from build123d import *

# Parameters (mm, degrees)
F0_W     = 35.56
F0_H     = 37.1792408654
F1_DEPTH = 17.4625
F3_DEPTH = 4.7625
F4_R     = 5.08
F5_R     = 5.08


# Not quite as in the source:
# - a length typed as a fraction of an inch, garbled in the dataset ("3 / 203.2 mm" for 3/8 in), is restored


with BuildPart() as f1:
    # F0 (on Top) → F1 (new body)
    with BuildSketch(Plane.XY):
        Rectangle(F0_W, F0_H)
    extrude(amount=F1_DEPTH)

    # F2 (on face) → F3 (cut)
    with BuildSketch(Plane.XY.offset(17.4625)):
        with BuildLine():
            Line((-12.7, -18.5896204327), (17.78, -18.5896204327))
            Line((17.78, -18.5896204327), (17.78, 13.5096204327))
            Line((17.78, 13.5096204327), (-8.89, 13.5096204327))
            ThreePointArc((-8.89, 13.5096204327), (-15.3940768363, 16.203697269), (-12.7, 9.6996204327))
            Line((-12.7, 9.6996204327), (-12.7, -18.5896204327))
        make_face()
    extrude(amount=-F3_DEPTH, mode=Mode.SUBTRACT)

    # F4
    f4_edges = [f1.edges().sort_by_distance(p)[0] for p in [
        (-12.7, 9.69962, 15.08125),
        (-8.89, 13.50962, 15.08125),
    ]]
    fillet(f4_edges, radius=F4_R)

    # F5
    f5_edges = [f1.edges().sort_by_distance(p)[0] for p in [
        (-17.78, 18.58962, 8.73125),
    ]]
    fillet(f5_edges, radius=F5_R)


solid = f1.part
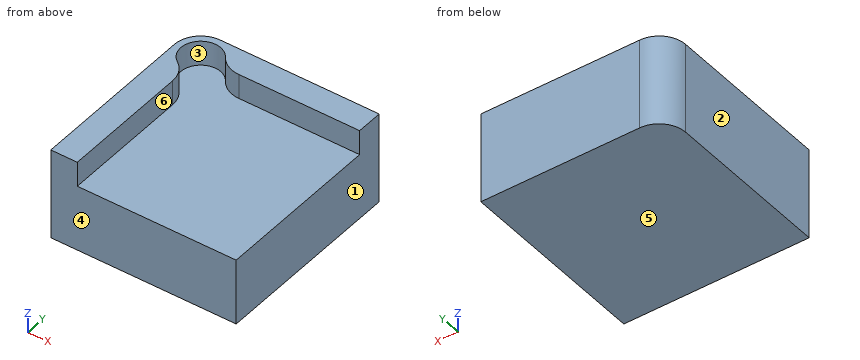
The listing builds one solid part. Answer for the finished solid, in the listing's coordinates (mm). Face numbers are marked on the shaded views. A direction names the side the tool comes from. Round coordinates to 2 decimals unless told otherwise and drop trailing zeros. Write each loop counter-clockwise with the first axis right and the second up, starting at its lowest first coordinate (ties: lowest second). Pieces come first, ordered by that corner, then holes. Notation, with made-up numbers: M 40,-4.75 L 70,-4.75 A12 cw 70,17.25 Z; hole C -19,29 d5. An arc over 180 degrees is marked long. Write each question's results on one line, items separated by ' | '. Start each with the question number.
(1) This flat-tipped pin is pushed along its axis until it touches: P1, Ø5, axis at x = 11.5, z = 16, coming from the -Y side. Where does it stop, or does it pass through?
(2) Find the intervals of material crossed by line 1 (Z direction, x = -8, y = -15.5); line 2 (X direction, y = 5.5, z = 13.5); line 3 (Y direction, x = 13, z = 15.25), in increasing order.
(3) For the marked faces 5 and 6, determine the directions among +Z, -Z, +X, -X, +Y, -Y from which every point of the face is accessible in a straight line to the end or side of a thin tool.
(4) The part is cut by section C-C, the plane y = 14. Write down the section's boundary in (x, z), and give its area (3 significant figures).
(5) Determine the mould class of the marked faces 1, 2, 3 and 4 for opening direction X: +X half, -X half, draft (parallel to the pull), parting line (faces both ways), or undercut.
(6) The part is cut by section A-A, the plane y = 2. Write down the section's boundary in (x, z).
(7) The part is cut by section B-B, the plane x = -14. Write down the section's boundary in (y, z), and give its area (3 significant figures).
Worked answers:
1) P1: stops at y = 13.51
2) line 1: z = 0 to 12.7 | line 2: x = -17.78 to -12.7 | line 3: y = 13.51 to 18.59
3) face 5: -Z, +X, -X, +Y, -Y | face 6: +Z, +X, -Y
4) outline: M -17.76,0 L 17.78,0 L 17.78,17.46 L -7.58,17.46 L -7.58,12.7 L -16.48,12.7 L -16.48,17.46 L -17.76,17.46 Z | area: 578 mm²
5) face 1: +X half | face 2: -X half | face 3: undercut | face 4: draft
6) outline: M -17.78,0 L 17.78,0 L 17.78,12.7 L -12.7,12.7 L -12.7,17.46 L -17.78,17.46 Z
7) outline: M -18.59,0 L 18.42,0 L 18.42,17.46 L 17.09,17.46 L 17.09,12.7 L 9.61,12.7 L 9.61,17.46 L -18.59,17.46 Z | area: 611 mm²
